from build123d import *

# Parameters (mm, degrees)
F0_R     = 25
F1_DEPTH = 3


# Not quite as in the source:
# - a feature of the source that left no trace in its solid (it failed there, or was rolled back) is left out


with BuildPart() as f1:
    # F0 (on Front) → F1 (new body)
    with BuildSketch(Plane.XZ):
        with BuildLine():
            Line((43.65, 50), (-43.65, 50))
            ThreePointArc((-43.65, 50), (-48.1401280605, 48.1401280605), (-50, 43.65))
            Line((-50, 43.65), (-50, -43.65))
            ThreePointArc((-50, -43.65), (-48.1401280605, -48.1401280605), (-43.65, -50))
            Line((-43.65, -50), (43.65, -50))
            ThreePointArc((43.65, -50), (48.1401280605, -48.1401280605), (50, -43.65))
            Line((50, -43.65), (50, 43.65))
            ThreePointArc((50, 43.65), (48.1401280605, 48.1401280605), (43.65, 50))
        make_face()
        Circle(F0_R, mode=Mode.SUBTRACT)
    extrude(amount=F1_DEPTH)


solid = f1.part
The listing builds one solid part. Answer for the finished solid, in the listing's coordinates (mm). Coordinates: 2 decimals unless noted, no trailing zeros. Loops run counter-clockwise (first coordinate to the right, second up) from the corner with the lowest first, then second, coordinate; pieces in that order, holes last.
1) Find section B-B on x = -20. Write down the section's boundary in (y, z).
2) Determine the mould class of faces 1 (the face through (-48.19, -1.48, -48.09)), 2 (the face through (-1, -1, -50)), 3 (the face through (50, -1, -1)), 4 (the face through (23.846, -1.479, 7.509)) for opening direction X: pulls with the +X half, pulls with the -X half, needs draft (parallel to the pull), parting line crosses it, or undercut.
3) Find the intervals of material crossed by L1, parallel to Z at x = 0, y = -0.55; L2, parallel to Z at x = 12, y = -0.6; L3, parallel to X at y = -1.35, z = -14.5, in increasing order.
4) A flat-ended cylindrical pin translates along its axis: pin 1 Ø12 at (x, z) = (15.5, -10) entering from +Y. Find the tip coordinate at first contact, or state that the pin passes through.
5) Find section A-A on z = 0. Write down the section's boundary in (x, y), then the cut area to 3 significant figures.
6) Find section C-C on y = -1.1. Write down the section's boundary in (x, z), then the cut area to 3 significant figures.
Values:
1. outline: (-3, -50) - (0, -50) - (0, -15) - (-3, -15) - close; (-3, 15) - (0, 15) - (0, 50) - (-3, 50) - close
2. face 1: pulls with the -X half
2. face 2: needs draft
2. face 3: pulls with the +X half
2. face 4: undercut
3. L1: z = -50 to -25, 25 to 50
3. L2: z = -50 to -21.93, 21.93 to 50
3. L3: x = -50 to -20.37, 20.37 to 50
4. pin 1: passes through
5. outline: (-50, -3) - (-25, -3) - (-25, 0) - (-50, 0) - close; (25, -3) - (50, -3) - (50, 0) - (25, 0) - close
5. area: 150 mm2
6. outline: (-50, -43.65) arc R6.35 ccw to (-43.65, -50) - (43.65, -50) arc R6.35 ccw to (50, -43.65) - (50, 43.65) arc R6.35 ccw to (43.65, 50) - (-43.65, 50) arc R6.35 ccw to (-50, 43.65) - close; hole circle Ø50 at (0, 0)
6. area: 8,000 mm2
